from build123d import *

# Parameters (mm, degrees)
SKETCH1_W           = 35
SKETCH1_H           = 20
BOSS_EXTRUDE1_DEPTH = 2
SKETCH3_R           = 1.5
CUT_EXTRUDE1_DEPTH  = 2
BOSS_EXTRUDE2_DEPTH = 2
SKETCH5_R           = 1.5
CUT_EXTRUDE2_DEPTH  = 2
SKETCH6_R           = 3.05
CUT_EXTRUDE3_DEPTH  = 1


with BuildPart() as part:
    # Sketch1 → Boss-Extrude1 (new body)
    with BuildSketch(Plane(origin=(0, 0, 0), x_dir=(0, 0, -1), z_dir=(1, 0, 0))):
        Rectangle(SKETCH1_W, SKETCH1_H)
    extrude(amount=BOSS_EXTRUDE1_DEPTH)

    # Sketch3 → Cut-Extrude1 (cut)
    with BuildSketch(Plane(origin=(2, 0, 0), x_dir=(0, 0, -1), z_dir=(1, 0, 0))):
        with Locations((10.5, 4)):
            Circle(SKETCH3_R)
        with Locations((10.5, -4)):
            Circle(SKETCH3_R)
        with Locations((-9.5, 4)):
            Circle(SKETCH3_R)
        with Locations((-9.5, -4)):
            Circle(SKETCH3_R)
    extrude(amount=-CUT_EXTRUDE1_DEPTH, mode=Mode.SUBTRACT)

    # Sketch4 → Boss-Extrude2 (add)
    with BuildSketch(Plane.XZ.offset(10)):
        Polygon((2, 7.5), (12, 11.642135624), (12, -15.428932188), (7, -17.5), (2, -17.5), align=None)
    extrude(amount=-BOSS_EXTRUDE2_DEPTH)

    # Sketch5 → Cut-Extrude2 (cut)
    with BuildSketch(Plane(origin=(0, -8, 0), x_dir=(1, 0, 0), z_dir=(0, 1, 0))):
        with Locations(Location((7, 12.717304889, 0), (0, 0, 270))):
            Circle(SKETCH5_R)
        with Locations(Location((7, -5.782695111, 0), (0, 0, 270))):
            Circle(SKETCH5_R)
    extrude(amount=-CUT_EXTRUDE2_DEPTH, mode=Mode.SUBTRACT)

    # Sketch6 → Cut-Extrude3 (cut)
    with BuildSketch(Plane(origin=(2, 0, 0), x_dir=(0, 0, -1), z_dir=(1, 0, 0))):
        with Locations((-9.5, 4)):
            Circle(SKETCH6_R)
        with Locations((-9.5, -4)):
            Circle(SKETCH6_R)
        with Locations((10.5, -4)):
            Circle(SKETCH6_R)
        with Locations((10.5, 4)):
            Circle(SKETCH6_R)
    extrude(amount=-CUT_EXTRUDE3_DEPTH, mode=Mode.SUBTRACT)


solid = part.part
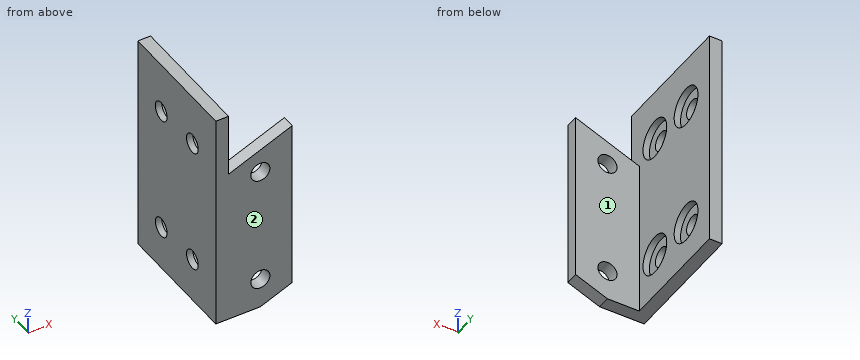
Here's how the part is built. I have some questions about the finished solid (model axes, mm). Face numbers are marked on the shaded views. A direction names the side the tool comes from. Coordinates: 2 decimals unless noted, no trailing zeros. Order: outer loops, then holes, each group sorted by start corner. A loop starts at its lowest first (then second) coordinate and runs counter-clockwise, first axis right, second up.
Item 1: I need wall thicknesses on line 1 (Y direction, x = 1.45, z = 9.5); line 2 (Y direction, x = 0.65, z = 9.5); line 3 (X direction, y = -1.5, z = 1). Which ranges of each line are inside material? Lowest first, please.
Result sheet:
line 1: y = -10 to -7.05, -0.95 to 0.95, 7.05 to 10
line 2: y = -10 to -5.5, -2.5 to 2.5, 5.5 to 10
line 3: x = 0 to 2
Item 2: If we section it at D-D on z = -1: List the corners of the cut face in (x, y) for me.
Result sheet:
outline: (0, -10) - (12, -10) - (12, -8) - (2, -8) - (2, 10) - (0, 10) - close
Item 3: For P1, Ø2, axis at x = 4, y = 4.5, coming from the -Z side; P2, Ø6, axis at y = 4, z = -5, coming from the +X side; P3, Ø4, axis at x = 7, z = -12.72, coming from the +Y side; P4, Ø3.5, axis at y = -4, z = 9.5, coming from the +X side, each with a flat end and sliding along its axis, tell me the tip position at first contact or that it passes through.
Result sheet:
P1: passes through
P2: stops at x = 2
P3: stops at y = -8
P4: stops at x = 1
Item 4: If we section it at C-C on z = 9.5: List the corners of the cut face in (x, y) for me, plus the area to 3 significant figures.
Result sheet:
outline: (0, -10) - (2, -10) - (2, -7.05) - (1, -7.05) - (1, -5.5) - (0, -5.5) - close; (0, -2.5) - (1, -2.5) - (1, -0.95) - (2, -0.95) - (2, 0.95) - (1, 0.95) - (1, 2.5) - (0, 2.5) - close; (0, 5.5) - (1, 5.5) - (1, 7.05) - (2, 7.05) - (2, 10) - (0, 10) - close; (6.83, -10) - (12, -10) - (12, -8) - (6.83, -8) - close
area: 32.1 mm2
Item 5: For the marked faces 1 and 2, which set-ups out of +Z, -Z, +X, -X, +Y, -Y let a thin tool reach every point of the face, with its end or its side?
Result sheet:
face 1: +Z, -Z, +X, +Y
face 2: +Z, -Z, +X, -X, -Y
Item 6: If we section it at A-A on z = -10.5: List the corners of the cut face in (x, y) for me.
Result sheet:
outline: (0, -10) - (12, -10) - (12, -8) - (2, -8) - (2, -7.05) - (1, -7.05) - (1, -5.5) - (0, -5.5) - close; (0, -2.5) - (1, -2.5) - (1, -0.95) - (2, -0.95) - (2, 0.95) - (1, 0.95) - (1, 2.5) - (0, 2.5) - close; (0, 5.5) - (1, 5.5) - (1, 7.05) - (2, 7.05) - (2, 10) - (0, 10) - close
Item 7: If we section it at B-B on y = 4: List the corners of the cut face in (x, z) for me.
Result sheet:
outline: (0, -17.5) - (2, -17.5) - (2, -13.55) - (1, -13.55) - (1, -12) - (0, -12) - close; (0, -9) - (1, -9) - (1, -7.45) - (2, -7.45) - (2, 6.45) - (1, 6.45) - (1, 8) - (0, 8) - close; (0, 11) - (1, 11) - (1, 12.55) - (2, 12.55) - (2, 17.5) - (0, 17.5) - close
